Can you work these out from the model? Positions are in its coordinate system, mm. A direction names the side the tool comes from. Coordinates: 2 decimals unless noted, no trailing zeros. Write each loop counter-clockwise with the first axis right and the second up, starting at its lowest first coordinate (ties: lowest second). Pieces come first, ordered by that corner, then holes. Notation, with made-up numbers: (67, -22) - (91, -22) arc R23 cw to (91, 1) - close; hole circle Ø9 at (31.25, 12). An arc over 180 degrees is marked (long way). Use one line per item in the form item = value. Start each with the question number.
(1) If we section it at A-A on x = 0: Please give me the cut outline in (y, z).
(2) Thinking about a two-plate mould opening in Z: for faces 4 (the face through (35, 1, 19)), 5 (the face through (1, 1, -35)), 6 (the face through (-42, 1, 3)), 7 (the face through (0.05, 1.48, 8.95)), which applies, pulls with the +Z half, pulls with the -Z half, needs draft (parallel to the pull), parting line crosses it, or undercut?
(3) If we section it at D-D on x = 44: Please give me the cut outline in (y, z), then the cut area to 4 significant figures.
(4) If we section it at C-C on x = -30.7: Please give me the cut outline in (y, z), then the cut area to 3 significant figures.
(5) For pin 1 Ø2 at (x, z) = (-30.7, 28.05) entering from -Y; pin 2 Ø1 at (y, z) = (1, 19) entering from +X; pin 3 Ø0.9 at (x, y) = (42, 1.5) entering from +Z, each with a flat end and sliding along its axis, tell me the tip position at first contact or that it passes through.
(6) If I drill on probe 1 along Z at (x, y) = (-30.7, 0.7); probe 2 along Z at (x, y) = (0, 2.3); probe 3 along X at (y, z) = (0.75, 10.5), over which ranges is the centre line in solid material (lowest first)? Write a range as from..to.
(7) If we section it at B-B on z = 9.95: Please give me the cut outline in (x, y).
(8) On a 3-axis mill with a long thin cutter (end or side, diameter ignored), from which of +Z, -Z, +X, -X, +Y, -Y can I reach the whole of each face in a straight line? I mean faces 1 (the face through (-0.479, 1.479, -31.155)), 2 (the face through (-35, 1, 19)), 3 (the face through (43, 1, 3)). Say none if no direction works.
Autodesk Inventor part; units mm, degrees
ref_plane "YZ Plane" through (0, 0, 0) normal (1, 0, 0) x (0, 1, 0)
ref_plane "XZ Plane" through (0, 0, 0) normal (0, 1, 0) x (-1, 0, 0)
ref_plane "XY Plane" through (0, 0, 0) normal (0, 0, 1) x (1, 0, 0)
sketch "Sketch1" plane through (0, 0, 0) normal (0, 1, 0) x (-1, 0, 0)
  line L0 (35, 35) -> (35, 3)
  line L1 (9, 3) -> (35, 3) construction
  line L2 (0, 3) -> (9, 3) construction
  line L3 (35, 3) -> (50, 3)
  line L4 (0, -35) -> (0, 35)
  line L5 (0, -35) -> (50, -35)
  line L6 (0, 35) -> (35, 35)
  line L7 (50, -35) -> (50, 3)
  line L8 (30.7, 28.05) -> (35, 28.05) construction
  line L9 (30.7, 28.05) -> (30.7, 9.95) construction
  line L10 (30.7, 9.95) -> (30.7, 3) construction
  circle A0 centre (30.7, 9.95) radius 1.25
  circle A1 centre (30.7, 28.05) radius 1.25
  line L11 (50, -16) -> (37.1975, -16) construction
  circle A2 centre (44, -3) radius 1.25
  arc A3 (0, -31.25) -> (0, -28.75) centre (0, -30) ccw
  arc A4 (0, 6.45) -> (0, 8.95) centre (0, 7.7) ccw
  arc A5 (0, 28.05) -> (0, 30.55) centre (0, 29.3) ccw
  line L12 (0, 29.3) -> (30.7, 29.3) construction
  point P0 (0, 0)
  point P1 (-50, 0)
  point P2 (0, 0)
  dimension "d26" = 2.5
  dimension "d6" = 32
  dimension "d9" = 26
  dimension "d10" = 9
  dimension "d11" = 50
  dimension "d12" = 70
  dimension "d14" = 4.3
  dimension "d15" = 18.1
  dimension "d20" = 6.95
  dimension "d25" = 2.5
  dimension "d32" = 2.5
  dimension "d33" = 2.5
  dimension "d35" = 2.5
  dimension "d36" = 2.5
  dimension "d37" = 2.25
  dimension "d38" = 6
  dimension "d39" = 5
  dimension "d40" = 6
extrude "Extrusion1" add sketch "Sketch1" along normal blind 3 contours L0 L3 L7 L5 L4 A3 A4 A5 L6 | A5 L4 | A4 L4 | L4 A3 | A0 | A1 | A2
extrude "Extrusion4" cut sketch "Sketch1" along normal through all contours A5 L4 | A4 L4 | L4 A3 | A0 | A1 | A2
mirror "Mirror1" about plane through (0, 0, 0) normal (1, 0, 0) of "Extrusion1", "Extrusion4"
properties part number "Podstawa"
Reported:
q1.outline = (0, -35) - (3, -35) - (3, -31.25) - (0, -31.25) - close; (0, -28.75) - (3, -28.75) - (3, 6.45) - (0, 6.45) - close; (0, 8.95) - (3, 8.95) - (3, 28.05) - (0, 28.05) - close; (0, 30.55) - (3, 30.55) - (3, 35) - (0, 35) - close
q2.face_4 = needs draft
q2.face_5 = pulls with the -Z half
q2.face_6 = pulls with the +Z half
q2.face_7 = undercut
q3.outline = (0, -35) - (3, -35) - (3, -4.25) - (0, -4.25) - close; (0, -1.75) - (3, -1.75) - (3, 3) - (0, 3) - close
q3.area = 106.5 mm2
q4.outline = (0, -35) - (3, -35) - (3, 8.7) - (0, 8.7) - close; (0, 11.2) - (3, 11.2) - (3, 26.8) - (0, 26.8) - close; (0, 29.3) - (3, 29.3) - (3, 35) - (0, 35) - close
q4.area = 195 mm2
q5.pin_1 = through
q5.pin_2 = 35
q5.pin_3 = 3
q6.probe_1 = -35..8.7, 11.2..26.8, 29.3..35
q6.probe_2 = -35..-31.25, -28.75..6.45, 8.95..28.05, 30.55..35
q6.probe_3 = -35..-31.82, -29.58..29.58, 31.82..35
q7.outline = (-35, 0) - (-31.95, 0) - (-31.95, 3) - (-35, 3) - close; (-29.45, 0) - (29.45, 0) - (29.45, 3) - (-29.45, 3) - close; (31.95, 0) - (35, 0) - (35, 3) - (31.95, 3) - close
q8.face_1 = +Y, -Y
q8.face_2 = +Z, -X, +Y, -Y
q8.face_3 = +Z, +X, +Y, -Y
